CAD build for the part. Positions are in the model's coordinates, mm. Face numbers are marked on the shaded views. Give positions to 0.01 mm unless a question says otherwise; leave off trailing zeros. Loops run counter-clockwise (first coordinate to the right, second up) from the corner with the lowest first, then second, coordinate; pieces in that order, holes last. Notation, with made-up numbers: (3.25, -39.75) - (57.25, -39.75) arc R30 cw to (57.25, -1.75) - close; hole circle Ø4 at (-32.5, -31). An arc over 180 degrees is marked (long way). Return JSON: item names as keys, results as strings.
Solid Edge part; units mm, degrees
sketch "Sketch1" plane through (0, 0, 0) normal (0, -1, 0) x (1, 0, 0)
  line L0 (-30, -30) -> (30, -30)
  line L1 (30, -30) -> (30, 30)
  line L2 (30, 30) -> (-30, 30)
  line L3 (-30, 30) -> (-30, -30)
  dimension "D1" = 30
extrude "Protrusion1" add sketch "Sketch1" along normal mid plane 12
fillet "Round_1" radius 5 4 edges at (30, 0, 30) (30, 0, -30) (-30, 0, -30) (-30, 0, 30)
hole "Hole_1" at (-22.5, -6, 22.5) direction (0, 1, 0) diameter 3.6 end up to next
hole "Hole1" at (22.5, -6, 22.5) direction (0, 1, 0) diameter 3.6 end up to next
hole "Hole2" at (22.5, -6, -22.5) direction (0, 1, 0) diameter 3.6 end up to next
hole "Hole3" at (-22.5, -6, -22.5) direction (0, 1, 0) diameter 3.6 end up to next
hole "Hole_5" at (0, -6, 0) direction (0, 1, 0) diameter 6 end up to next counterbore diameter 22.5 counterbore depth 2
hole "Hole_6" at (0, 6, 21.9203) direction (0, -1, 0) diameter 3.6 end up to next counterbore diameter 6.5 counterbore depth 3.5
hole "Hole4" at (-21.9203, 6, 0) direction (0, -1, 0) diameter 3.6 end up to next counterbore diameter 6.5 counterbore depth 3.5
hole "Hole5" at (0, 6, -21.9203) direction (0, -1, 0) diameter 3.6 end up to next counterbore diameter 6.5 counterbore depth 3.5
hole "Hole6" at (21.9203, 6, 0) direction (0, -1, 0) diameter 3.6 end up to next counterbore diameter 6.5 counterbore depth 3.5
properties material "Polyethylene, low density"
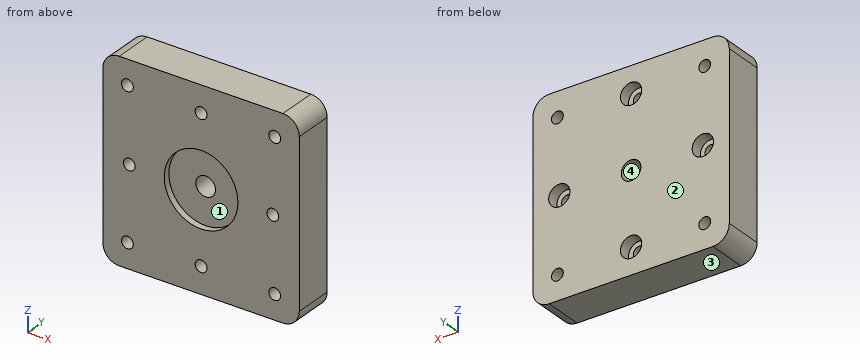
1. Cut at C-C, the plane y = 3.5. Give the number of separate pieces and of enclosed holes in the cut face, plus the area to 3 significant figures.
Values follow:
{"separate pieces": "1", "enclosed holes": "9", "area": "3,380 mm²"}
2. Drill centre lines: probe 1 along X at (y, z) = (5.25, 0); probe 2 along X at (y, z) = (-4.65, 0); probe 3 along X at (y, z) = (-1.25, -24). Where is each one in solid material? Low to high.
Values follow:
{"probe 1": "x = -30 to -25.17, -18.67 to -3, 3 to 18.67, 25.17 to 30", "probe 2": "x = -30 to -23.72, -20.12 to -11.25, 11.25 to 20.12, 23.72 to 30", "probe 3": "x = -30 to -23.49, -21.51 to 21.51, 23.49 to 30"}
3. Drop a flat-ended pin along its axis: P1, Ø4.5, axis at x = -21.92, z = 0, coming from the +Y side. Give the stop position or say it passes through.
Values follow:
{"P1": "stops at y = 2.5"}
4. Cut at D-D, the plane x = -6.5. Write the cut outline in (y, z), plus the area to 3 significant figures.
Values follow:
{"outline": "(-6, -30) - (6, -30) - (6, 30) - (-6, 30) - (-6, 9.18) - (-4, 9.18) - (-4, -9.18) - (-6, -9.18) - close", "area": "683 mm²"}
5. Pull direction Z, two halves, no side cores. Call the marked faces 1, 2, 3 and 4: +Z half, -Z half, draft (parallel to the pull), parting line (faces both ways), or undercut.
Values follow:
{"face 1": "undercut", "face 2": "draft", "face 3": "-Z half", "face 4": "undercut"}
6. Cut at B-B, the plane z = 0. Write the cut outline in (x, y).
Values follow:
{"outline": "(-30, -6) - (-23.72, -6) - (-23.72, 2.5) - (-25.17, 2.5) - (-25.17, 6) - (-30, 6) - close; (-20.12, -6) - (-11.25, -6) - (-11.25, -4) - (-3, -4) - (-3, 6) - (-18.67, 6) - (-18.67, 2.5) - (-20.12, 2.5) - close; (3, -4) - (11.25, -4) - (11.25, -6) - (20.12, -6) - (20.12, 2.5) - (18.67, 2.5) - (18.67, 6) - (3, 6) - close; (23.72, -6) - (30, -6) - (30, 6) - (25.17, 6) - (25.17, 2.5) - (23.72, 2.5) - close"}
7. Cut at A-A, the plane x = 0. Write the cut outline in (y, z), plus the area to 3 significant figures.
Values follow:
{"outline": "(-6, -30) - (6, -30) - (6, -25.17) - (2.5, -25.17) - (2.5, -23.72) - (-6, -23.72) - close; (-6, -20.12) - (2.5, -20.12) - (2.5, -18.67) - (6, -18.67) - (6, -3) - (-4, -3) - (-4, -11.25) - (-6, -11.25) - close; (-6, 11.25) - (-4, 11.25) - (-4, 3) - (6, 3) - (6, 18.67) - (2.5, 18.67) - (2.5, 20.12) - (-6, 20.12) - close; (-6, 23.72) - (2.5, 23.72) - (2.5, 25.17) - (6, 25.17) - (6, 30) - (-6, 30) - close", "area": "508 mm²"}
